Geometry: final body of the model. Coordinates: model frame, mm. Face numbers are marked on the shaded views. A direction names the side the tool comes from. Round coordinates to 2 decimals unless told otherwise and drop trailing zeros. Loops run counter-clockwise (first coordinate to the right, second up) from the corner with the lowest first, then second, coordinate; pieces in that order, holes last. Notation, with made-up numbers: (15, 77) - (32, 77) arc R19 ccw to (32, 91) - close; hole circle Ø3 at (38.5, -17). An arc over 180 degrees is marked (long way). Return JSON: item names as keys, results as strings. Group by question number.
1. Set-up query: the marked faces 1, 2, 3 and 4. Return all of +Z, -Z, +X, -X, +Y, -Y with unobstructed straight access to the full face (end or side cutting, diameter ignored); none if empty.
2. Draft query along Z for the marked faces 5, 6, 7 and 8. Return one class per face: +Z half, -Z half, draft (parallel to the pull), parting line (faces both ways), or undercut.
3. Material intervals for probe 1 along X at (y, z) = (-1, 0); probe 2 along Y at (x, z) = (-22.5, 4.5); probe 3 along X at (y, z) = (-7.25, 3.5), sorted ascending.
4. Section C-C on z = 6.75. Return loops of the section in (x, y).
5. Section D-D on x = 7.5. Return loops of the section in (y, z), and give its area (3 significant figures).
6. Section B-B on x = 37.5. Return loops of the section in (y, z), and give its area (3 significant figures).
7. Section A-A on y = 5. Count the separate pieces of the cut face and the enclosed holes in it, and give its area (3 significant figures).
8. First-contact query: pin 1 Ø1 at (y, z) = (-3, -4.5) entering from -X; pin 2 Ø1.5 at (x, y) = (-33.5, -2.5) entering from -Z; pin 3 Ø6.5 at (x, z) = (-7.5, 0) entering from +Y; pin 4 Ø1.2 at (y, z) = (4.5, 0.5) entering from +X. Flat tips, straight axial feed; report the tip coordinate or a pass-through.
from build123d import *

# Parameters (mm, degrees)
SKETCH2_W           = 15
SKETCH2_H           = 15
SKETCH2_W_2         = 30
SKETCH2_R           = 4.15
BOSS_EXTRUDE1_DEPTH = 10
SKETCH2_3_W         = 15
SKETCH2_3_H         = 15
SKETCH2_3_W_2       = 30
SKETCH2_3_R         = 4.15
BOSS_EXTRUDE2_DEPTH = 10
SKETCH4_R           = 1.6
CUT_EXTRUDE1_DEPTH  = 16
CUT_EXTRUDE2_START  = -6.25
SKETCH4_3_R         = 1.6
CUT_EXTRUDE2_DEPTH  = 2.5
SKETCH5_W           = 15
SKETCH5_H           = 15
BOSS_EXTRUDE3_DEPTH = 5
CUT_EXTRUDE3_REACH  = 22
SKETCH6_R           = 1.6
SKETCH7_R           = 4.15
CUT_EXTRUDE4_DEPTH  = 8


with BuildPart() as part:
    # Sketch2 → Boss-Extrude1 (new body)
    with BuildSketch(Plane(origin=(0, 0, 0), x_dir=(1, 0, 0), z_dir=(0, 1, 0))):
        with Locations((-22.5, 0)):
            Rectangle(SKETCH2_W, SKETCH2_H)
        Rectangle(SKETCH2_W_2, SKETCH2_H)
        with Locations((7.5, 0)):
            Circle(SKETCH2_R, mode=Mode.SUBTRACT)
        with Locations((-7.5, 0)):
            Circle(SKETCH2_R, mode=Mode.SUBTRACT)
        with Locations((22.5, 0)):
            Rectangle(SKETCH2_W, SKETCH2_H)
    extrude(amount=BOSS_EXTRUDE1_DEPTH)

    # Sketch2_3 → Boss-Extrude2 (add)
    with BuildSketch(Plane(origin=(0, 0, 0), x_dir=(1, 0, 0), z_dir=(0, 1, 0))):
        with Locations((-22.5, 0)):
            Rectangle(SKETCH2_3_W, SKETCH2_3_H)
        Rectangle(SKETCH2_3_W_2, SKETCH2_3_H)
        with Locations((7.5, 0)):
            Circle(SKETCH2_3_R, mode=Mode.SUBTRACT)
        with Locations((-7.5, 0)):
            Circle(SKETCH2_3_R, mode=Mode.SUBTRACT)
        with Locations((-7.5, 0)):
            Circle(SKETCH2_3_R)
        with Locations((7.5, 0)):
            Circle(SKETCH2_3_R)
        with Locations((22.5, 0)):
            Rectangle(SKETCH2_3_W, SKETCH2_3_H)
    extrude(amount=-BOSS_EXTRUDE2_DEPTH)

    # Sketch4 → Cut-Extrude1 (cut, through all)
    with BuildSketch(Plane.XY.offset(7.5)):
        with Locations((-22.5, -5)):
            Circle(SKETCH4_R)
        with Locations((-22.5, 5)):
            Circle(SKETCH4_R)
        with Locations((22.5, 5)):
            Circle(SKETCH4_R)
        with Locations((22.5, -5)):
            Circle(SKETCH4_R)
    extrude(amount=-CUT_EXTRUDE1_DEPTH, mode=Mode.SUBTRACT)

    # Sketch4_3 → Cut-Extrude2 (cut)
    with BuildSketch(Plane.XY.offset(7.5).offset(CUT_EXTRUDE2_START)):
        Polygon((-22.5, 8.435234102), (-25.475, 6.717617051), (-25.475, 3.282382949), (-22.5, 1.564765898), (-19.525, 3.282382949), (-19.525, 6.717617051), align=None)
        with Locations((-22.5, 5)):
            Circle(SKETCH4_3_R, mode=Mode.SUBTRACT)
        Polygon((22.5, 8.435234102), (19.525, 6.717617051), (19.525, 3.282382949), (22.5, 1.564765898), (25.475, 3.282382949), (25.475, 6.717617051), align=None)
        with Locations((22.5, 5)):
            Circle(SKETCH4_3_R, mode=Mode.SUBTRACT)
        Polygon((-22.5, -8.435234102), (-19.525, -6.717617051), (-19.525, -3.282382949), (-22.5, -1.564765898), (-25.475, -3.282382949), (-25.475, -6.717617051), align=None)
        with Locations((-22.5, -5)):
            Circle(SKETCH4_3_R, mode=Mode.SUBTRACT)
        Polygon((22.5, -8.435234102), (25.475, -6.717617051), (25.475, -3.282382949), (22.5, -1.564765898), (19.525, -3.282382949), (19.525, -6.717617051), align=None)
        with Locations((22.5, -5)):
            Circle(SKETCH4_3_R, mode=Mode.SUBTRACT)
    extrude(amount=-CUT_EXTRUDE2_DEPTH, mode=Mode.SUBTRACT)

    # Sketch5 → Boss-Extrude3 (add)
    with BuildSketch(Plane.XZ.offset(10)):
        with Locations((-37.5, 0)):
            Rectangle(SKETCH5_W, SKETCH5_H)
        with Locations((37.5, 0)):
            Rectangle(SKETCH5_W, SKETCH5_H)
    extrude(amount=-BOSS_EXTRUDE3_DEPTH)

    # Sketch6 → Cut-Extrude3 (cut, up to next)
    with BuildSketch(Plane.XZ.offset(10), mode=Mode.PRIVATE) as cut_extrude3_sk1:
        with Locations((-37.5, 0)):
            Circle(SKETCH6_R)
    cut_extrude3_tool1 = extrude(cut_extrude3_sk1.sketch, amount=-CUT_EXTRUDE3_REACH, mode=Mode.PRIVATE) & part.part
    add(cut_extrude3_tool1.solids().sort_by_distance((-37.5, -10, 0))[0], mode=Mode.SUBTRACT)
    # Sketch6 → Cut-Extrude3 (cut, up to next)
    with BuildSketch(Plane.XZ.offset(10), mode=Mode.PRIVATE) as cut_extrude3_sk2:
        with Locations((37.5, 0)):
            Circle(SKETCH6_R)
    cut_extrude3_tool2 = extrude(cut_extrude3_sk2.sketch, amount=-CUT_EXTRUDE3_REACH, mode=Mode.PRIVATE) & part.part
    add(cut_extrude3_tool2.solids().sort_by_distance((37.5, -10, 0))[0], mode=Mode.SUBTRACT)

    # Sketch7 → Cut-Extrude4 (cut)
    with BuildSketch(Plane(origin=(0, 0, 0), x_dir=(1, 0, 0), z_dir=(0, 1, 0))):
        with Locations((-7.5, 0)):
            Circle(SKETCH7_R)
        with Locations((7.5, 0)):
            Circle(SKETCH7_R)
    extrude(amount=-CUT_EXTRUDE4_DEPTH, mode=Mode.SUBTRACT)


solid = part.part
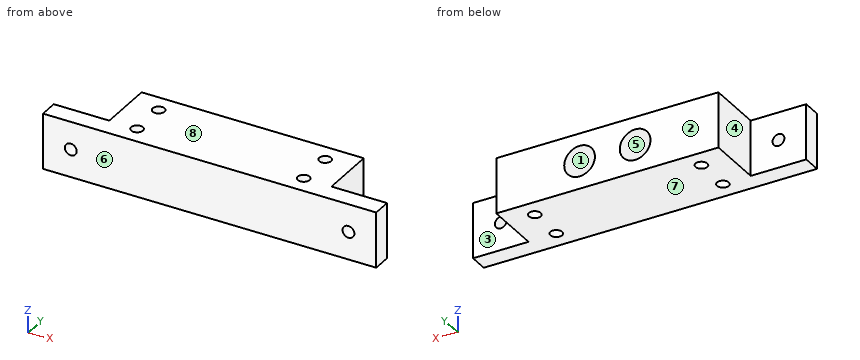
Taken from the geometry:
{
 "1": {"face 1": "+Y", "face 2": "+Z, -Z, +X, -X, +Y", "face 3": "+Z, -Z, +X, +Y", "face 4": "+Z, -Z, -X, +Y"},
 "2": {"face 5": "undercut", "face 6": "draft", "face 7": "-Z half", "face 8": "+Z half"},
 "3": {"probe 1": "-30 to -11.65, -3.35 to 3.35, 11.65 to 30", "probe 2": "-10 to -6.6, -3.4 to 3.4, 6.6 to 10", "probe 3": "-45 to -9.73, -5.27 to 5.27, 9.73 to 45"},
 "4": {"outline": "(-45, -10) - (45, -10) - (45, -5) - (30, -5) - (30, 10) - (-30, 10) - (-30, -5) - (-45, -5) - close; hole circle Ø3.2 at (-22.5, -5); hole circle Ø3.2 at (-22.5, 5); hole circle Ø3.2 at (22.5, -5); hole circle Ø3.2 at (22.5, 5)"},
 "5": {"outline": "(-10, -7.5) - (10, -7.5) - (10, -4.15) - (-8, -4.15) - (-8, 4.15) - (10, 4.15) - (10, 7.5) - (-10, 7.5) - close", "area": "151 mm2"},
 "6": {"outline": "(-10, -7.5) - (-5, -7.5) - (-5, -1.6) - (-10, -1.6) - close; (-10, 1.6) - (-5, 1.6) - (-5, 7.5) - (-10, 7.5) - close", "area": "59.0 mm2"},
 "7": {"separate pieces": "3", "enclosed holes": "2", "area": "682 mm2"},
 "8": {"pin 1": "x = -30", "pin 2": "through", "pin 3": "y = -8", "pin 4": "x = 30"}
}
